Part model, mm, in its own coordinate system. Give positions to 0.01 mm unless a question says otherwise; leave off trailing zeros. Loops run counter-clockwise (first coordinate to the right, second up) from the corner with the lowest first, then second, coordinate; pieces in that order, holes last. Notation, with made-up numbers: M 13.25,5.5 L 17.25,5.5 A34 cw 17.25,40.5 Z; hole C -2,19 d4. An arc over 180 degrees is marked long. Answer in a Markdown table with one row per item.
from build123d import *

# Parameters (mm, degrees)
F0_W     = 125
F0_H     = 40
F0_R     = 1.75
F1_DEPTH = 2
F2_R     = 1.5
F3_R     = 3


# Not quite as in the source:
# - a feature names something its author has since deleted; it is built from what else it names


with BuildPart() as f1:
    # F0 (on Front) → F1 (new body)
    with BuildSketch(Plane.XZ):
        Rectangle(F0_W, F0_H)
        with Locations((-55, -15)):
            Circle(F0_R, mode=Mode.SUBTRACT)
        with Locations((55, -15)):
            Circle(F0_R, mode=Mode.SUBTRACT)
        with BuildLine():
            Line((-57.5, 2), (-52, 2))
            Line((-52, 2), (-52, 7.5))
            ThreePointArc((-52, 7.5), (-50, 9.5), (-48, 7.5))
            Line((-48, 7.5), (-48, 2))
            Line((-48, 2), (-42.5, 2))
            ThreePointArc((-42.5, 2), (-40.5, 0), (-42.5, -2))
            Line((-42.5, -2), (-48, -2))
            Line((-48, -2), (-48, -7.5))
            ThreePointArc((-48, -7.5), (-50, -9.5), (-52, -7.5))
            Line((-52, -7.5), (-52, -2))
            Line((-52, -2), (-57.5, -2))
            ThreePointArc((-57.5, -2), (-59.5, 0), (-57.5, 2))
        make_face(mode=Mode.SUBTRACT)
        with Locations((-55, 15)):
            Circle(F0_R, mode=Mode.SUBTRACT)
        Circle(F0_R, mode=Mode.SUBTRACT)
        with BuildLine():
            Line((42.5, 2), (48, 2))
            Line((48, 2), (48, 7.5))
            ThreePointArc((48, 7.5), (50, 9.5), (52, 7.5))
            Line((52, 7.5), (52, 2))
            Line((52, 2), (57.5, 2))
            ThreePointArc((57.5, 2), (59.5, 0), (57.5, -2))
            Line((57.5, -2), (52, -2))
            Line((52, -2), (52, -7.5))
            ThreePointArc((52, -7.5), (50, -9.5), (48, -7.5))
            Line((48, -7.5), (48, -2))
            Line((48, -2), (42.5, -2))
            ThreePointArc((42.5, -2), (40.5, 0), (42.5, 2))
        make_face(mode=Mode.SUBTRACT)
        with Locations((55, 15)):
            Circle(F0_R, mode=Mode.SUBTRACT)
    extrude(amount=F1_DEPTH)

    # F2
    f2_edges = [f1.edges().sort_by_distance(p)[0] for p in [
        (-62.5, -1, 20),
        (62.5, -1, 20),
        (-62.5, -1, -20),
        (62.5, -1, -20),
    ]]
    fillet(f2_edges, radius=F2_R)

    # F3
    f3_edges = [f1.edges().sort_by_distance(p)[0] for p in [
        (-48, -1, 2),
        (-52, -1, 2),
        (-52, -1, -2),
        (-48, -1, -2),
        (52, -1, 2),
        (48, -1, 2),
        (48, -1, -2),
        (52, -1, -2),
    ]]
    fillet(f3_edges, radius=F3_R)


solid = f1.part
(1) Saw through at D-D (y = -0.75). Give the number of separate pieces and of enclosed holes in the cut face, plus the area to 3 significant figures.
Recorded:
| item | result |
|---|---|
| separate pieces | 1 |
| enclosed holes | 7 |
| area | 4,680 mm^2 |
(2) Saw through at A-A (z = 0). Write the cut outline in (x, y), plus the area to 3 significant figures.
Recorded:
| item | result |
|---|---|
| outline | M -62.5,-2 L -59.5,-2 L -59.5,0 L -62.5,0 Z; M -40.5,-2 L -1.75,-2 L -1.75,0 L -40.5,0 Z; M 1.75,-2 L 40.5,-2 L 40.5,0 L 1.75,0 Z; M 59.5,-2 L 62.5,-2 L 62.5,0 L 59.5,0 Z |
| area | 167 mm^2 |
(3) Pull direction X, two halves, no side cores. Call faces 1 (the face through (-1, -1, 20)), 2 (the face through (52, -1, 6)), 3 (the face through (-62.5, -1, 0)): +X half, -X half, draft (parallel to the pull), parting line (faces both ways), or undercut.
Recorded:
| item | result |
|---|---|
| face 1 | draft |
| face 2 | undercut |
| face 3 | -X half |
(4) Saw through at C-C (z = -15). Write the cut outline in (x, y), plus the area to 3 significant figures.
Recorded:
| item | result |
|---|---|
| outline | M -62.5,-2 L -56.75,-2 L -56.75,0 L -62.5,0 Z; M -53.25,-2 L 53.25,-2 L 53.25,0 L -53.25,0 Z; M 56.75,-2 L 62.5,-2 L 62.5,0 L 56.75,0 Z |
| area | 236 mm^2 |
(5) Drill centre lines: line 1 along Z through (x, y) = (-55, -0.85); line 2 along Z through (x, y) = (43.5, -0.35); line 3 along Z through (x, y) = (0, -1). Where is each one in solid material? Low to high.
Recorded:
| item | result |
|---|---|
| line 1 | z = -20 to -16.75, -13.25 to -2, 2 to 13.25, 16.75 to 20 |
| line 2 | z = -20 to -2, 2 to 20 |
| line 3 | z = -20 to -1.75, 1.75 to 20 |
(6) Saw through at B-B (x = 0). Write the cut outline in (y, z).
Recorded:
| item | result |
|---|---|
| outline | M -2,-20 L 0,-20 L 0,-1.75 L -2,-1.75 Z; M -2,1.75 L 0,1.75 L 0,20 L -2,20 Z |
